Autodesk Inventor part; units mm, degrees
ref_plane "YZ Plane" through (0, 0, 0) normal (1, 0, 0) x (0, 1, 0)
ref_plane "XZ Plane" through (0, 0, 0) normal (0, 1, 0) x (-1, 0, 0)
ref_plane "XY Plane" through (0, 0, 0) normal (0, 0, 1) x (1, 0, 0)
sketch "Esquisse1" plane through (0, 0, 0) normal (0, 1, 0) x (-1, 0, 0)
  circle A0 centre (0, 0) radius 20
  dimension "d0" = 40
extrude "Extrusion1" add sketch "Esquisse1" along normal blind 20
sketch "Esquisse2" plane through (0, 0, 0) normal (0, -1, 0) x (1, 0, 0)
  circle A0 centre (0, 0) radius 20
  circle A1 centre (0, 0) radius 17
  dimension "d3" = 3
extrude "Extrusion2" cut sketch "Esquisse2" against normal blind 15
sketch "Esquisse3" plane through (0, 0, 0) normal (0, -1, 0) x (1, 0, 0)
  circle A0 centre (0, 0) radius 17
  circle A1 centre (0, 0) radius 14
  dimension "d6" = 3
extrude "Extrusion3" cut sketch "Esquisse3" against normal blind 15 contours A1
sketch "Esquisse4" plane through (0, 15, 0) normal (0, -1, 0) x (1, 0, 0)
  circle A0 centre (0, 0) radius 14
  circle A1 centre (0, 0) radius 5
  circle A2 centre (0, 11) radius 1.75
  circle A3 centre (0, -11) radius 1.75
  dimension "d9" = 10
  dimension "d10" = 3.5
  dimension "d11" = 3.5
  dimension "d12" = 11
  dimension "d13" = 11
extrude "Extrusion4" cut sketch "Esquisse4" against normal through all contours A1 | A2 | A3
equation "\"d11\" = d10"
equation "\"d13\" = d12"
properties part number "Bouchon PVC" material "PVC, non plastifié"
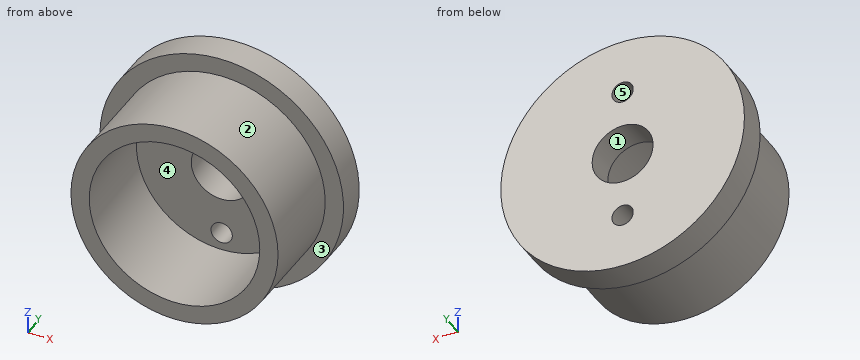
The model under review builds one solid part; all positions refer to its coordinate system, in mm. Face numbers are marked on the shaded views. A direction names the side the tool comes from. Coordinates: 2 decimals unless noted, no trailing zeros. Write each loop counter-clockwise with the first axis right and the second up, starting at its lowest first coordinate (ties: lowest second). Pieces come first, ordered by that corner, then holes. Notation, with made-up numbers: (8.5, 37) - (20.5, 37) arc R21 cw to (20.5, 62) - close; hole circle Ø6 at (75, -7). An arc over 180 degrees is marked (long way). Answer as CSV lines item,"result".
(1) For line 1 along Z through (x, y) = (0, 16.15); line 2 along Y through (x, z) = (-2, -10); line 3 along X through (y, z) = (1.25, 8), list the stretches that pass through material, from the lowest coordinate up. Write a range as [from, to].
Data:
line 1,"z = [-20, -12.75], [-9.25, -5], [5, 9.25], [12.75, 20]"
line 2,"y = [15, 20]"
line 3,"x = [-15, -11.49], [11.49, 15]"
(2) We need section D-D (x = 7.5). Give the boundary of the cut face in (y, z), plus the area to 3 significant figures.
Data:
outline,"(0, -15.26) - (15, -15.26) - (15, -18.54) - (20, -18.54) - (20, 18.54) - (15, 18.54) - (15, 15.26) - (0, 15.26) - (0, 11.82) - (15, 11.82) - (15, -11.82) - (0, -11.82) - close"
area,"288 mm2"
(3) Clearance check with flat-ended pins moving along their axes: pin 1 Ø2 at (y, z) = (7, 14) entering from +X; pin 2 Ø4 at (x, z) = (0, 11) entering from -Y; pin 3 Ø4 at (y, z) = (9.5, -10) entering from +X. State where each tip first meets the part, or that it passes through.
Data:
pin 1,"stops at x = 10.95"
pin 2,"stops at y = 15"
pin 3,"stops at x = 15"
(4) We need section A-A (x = 0). Give the boundary of the cut face in (y, z).
Data:
outline,"(0, -17) - (15, -17) - (15, -20) - (20, -20) - (20, -12.75) - (15, -12.75) - (15, -14) - (0, -14) - close; (0, 14) - (15, 14) - (15, 12.75) - (20, 12.75) - (20, 20) - (15, 20) - (15, 17) - (0, 17) - close; (15, -9.25) - (20, -9.25) - (20, -5) - (15, -5) - close; (15, 5) - (20, 5) - (20, 9.25) - (15, 9.25) - close"
(5) Tool access review of the marked faces 4 and 5: name each direction out of +Z, -Z, +X, -X, +Y, -Y from which nothing blocks a thin tool from reaching the whole face with its end or side.
Data:
face 4,"-Y"
face 5,"+Y, -Y"
(6) We need section C-C (y = 12.5). Give the boundary of the cut face in (x, z), plus the area to 3 significant figures.
Data:
outline,"circle Ø34 at (0, 0); hole circle Ø28 at (0, 0)"
area,"292 mm2"
(7) Mouldability with a two-part tool opening along X and no side actions: class the marked faces 1, 2 and 3 as pulls with the +X half, pulls with the -X half, needs draft (parallel to the pull), parting line crosses it, or undercut.
Data:
face 1,"undercut"
face 2,"parting line crosses it"
face 3,"needs draft"
(8) We need section B-B (z = 0). Give the boundary of the cut face in (x, y), plus the area to 3 significant figures.
Data:
outline,"(-20, 15) - (-17, 15) - (-17, 0) - (-14, 0) - (-14, 15) - (-5, 15) - (-5, 20) - (-20, 20) - close; (5, 15) - (14, 15) - (14, 0) - (17, 0) - (17, 15) - (20, 15) - (20, 20) - (5, 20) - close"
area,"240 mm2"
